Could you check a few things on this model? Use its own coordinates, in mm. A direction names the side the tool comes from. Give positions to 0.01 mm unless a question says otherwise; leave off trailing zeros. Loops run counter-clockwise (first coordinate to the right, second up) from the corner with the lowest first, then second, coordinate; pieces in that order, holes last. Notation, with made-up numbers: (51, -19.5) -> (85, -19.5) arc R22 ccw to (85, 18.5) -> close; hole circle Ø11 at (5, -12). An arc over 180 degrees is marked (long way). Write item = value, one per line. Start each with the question number.
1) I want a section at C-C (z = 33). List the corners of the cut face in (x, y) for me, and give its area (3 significant figures).
2) On a 3-axis mill with a long thin cutter (end or side, diameter ignored), from which of +Z, -Z, +X, -X, +Y, -Y can I reach the whole of each face in a straight line? I mean faces 1 (the face through (-32, 0, 19.05)), 2 (the face through (-11, -25.4, 30)). Say none if no direction works.
3) I need wall thicknesses on probe 1 along X at (y, z) = (7.5, 49); probe 2 along Z at (x, y) = (-29, -21) (3 decimals); probe 3 along Z at (x, y) = (-23.5, 15.5) (3 decimals). Which ranges of each line are inside material? Lowest first, please. Write a range as from..to.
4) I want a section at B-B (x = -26). List the corners of the cut face in (y, z) for me (3 decimals).
5) I want a section at A-A (y = 9). List the corners of the cut face in (x, z) for me (3 decimals).
6) I'm going to push flat-ended pins straight in: pin 1 Ø2 at (y, z) = (-1.5, 29) entering from -X; pin 2 Ø14 at (x, y) = (-29, -8.5) entering from +Z; pin 3 Ø6 at (y, z) = (18.5, 26.5) entering from -X. Where does each tip first touch, or does it pass through?
from build123d import *

# Parameters (mm, degrees)
BOSS_EXTRUDE1_DEPTH = 3.175
SKETCH2_W           = 12.7
SKETCH2_H           = 50.8
BOSS_EXTRUDE2_DEPTH = 31.75
FILLET1_R           = 12.7


with BuildPart() as part:
    # Sketch1 → Boss-Extrude1 (new body)
    with BuildSketch(Plane.XY.offset(15.875)):
        Polygon((-38.1, 25.4), (-38.1, -25.4), (-25.4, -25.4), (0, -25.4), (0, 25.4), align=None)
    extrude(amount=BOSS_EXTRUDE1_DEPTH)

    # Sketch2 → Boss-Extrude2 (add)
    with BuildSketch(Plane.XY.offset(50.8)):
        with Locations((-6.35, 0)):
            Rectangle(SKETCH2_W, SKETCH2_H)
    extrude(amount=-BOSS_EXTRUDE2_DEPTH)

    # Fillet1
    fillet1_edges = [part.edges().sort_by_distance(p)[0] for p in [
        (-12.7, 0, 19.05),
    ]]
    fillet(fillet1_edges, radius=FILLET1_R)


solid = part.part
Answer list:
q1.outline = (-12.7, -25.4) -> (0, -25.4) -> (0, 25.4) -> (-12.7, 25.4) -> close
q1.area = 645 mm^2
q2.face_1 = +Z, -X, +Y, -Y
q2.face_2 = +Z, -Z, +X, -X, -Y
q3.probe_1 = -12.7..0
q3.probe_2 = 15.875..19.05
q3.probe_3 = 15.875..19.193
q4.outline = (-25.4, 15.875) -> (25.4, 15.875) -> (25.4, 19.05) -> (-25.4, 19.05) -> close
q5.outline = (-38.1, 15.875) -> (0, 15.875) -> (0, 50.8) -> (-12.7, 50.8) -> (-12.7, 31.75) arc R12.7 cw to (-25.4, 19.05) -> (-38.1, 19.05) -> close
q6.pin_1 = -13.27
q6.pin_2 = 19.51
q6.pin_3 = -15.74
